```python
from build123d import *

# Parameters (mm, degrees)
PAD001_DEPTH         = 8
SKETCH004_R          = 1.6
POCKET001_DEPTH      = 5.301
POCKET001_DEPTH_BACK = 3.3011
SKETCH_W             = 17.3
SKETCH_H             = 12
SKETCH_R             = 1.5
SKETCH_R_2           = 1.6
PAD_DEPTH            = 5
SKETCH001_W          = 14
SKETCH001_H          = 12
SKETCH001_R          = 2.5
SKETCH001_R_2        = 1
POCKET_DEPTH         = 3.001
FILLET_R             = 3


with BuildPart() as clipbody:
    # Sketch003 → Pad001 (new body)
    with BuildSketch(Plane.XZ):
        with BuildLine():
            Line((0, -5.3), (-12, -5.3))
            Line((-12, -2.8), (-12, -5.3))
            Line((-1.746425, -2.8), (-12, -2.8))
            ThreePointArc((-1.746425, -2.8), (3.3, 0), (-1.746425, 2.8))
            Line((-1.746425, 2.8), (-12, 2.8))
            Line((-12, 2.8), (-12, 3.3001))
            Line((5.3, 3.3001), (-12, 3.3001))
            Line((5.3, 0), (5.3, 3.3001))
            ThreePointArc((0, -5.3), (3.747666, -3.747666), (5.3, 0))
        make_face()
    extrude(amount=-PAD001_DEPTH)

    # Sketch004 → Pocket001 (cut, two sides)
    with BuildSketch(Plane.XY) as pocket001_sk:
        with Locations((-9.5, 4)):
            Circle(SKETCH004_R)
    extrude(amount=-POCKET001_DEPTH, mode=Mode.SUBTRACT)
    extrude(pocket001_sk.sketch, amount=POCKET001_DEPTH_BACK, mode=Mode.SUBTRACT)


with BuildPart() as part_refined:
    # Sketch → Pad (new body)
    with BuildSketch(Plane.XY):
        with Locations((8.65, 6)):
            Rectangle(SKETCH_W, SKETCH_H)
        with Locations((9, 6)):
            Circle(SKETCH_R, mode=Mode.SUBTRACT)
        with Locations((2.5, 4)):
            Circle(SKETCH_R_2, mode=Mode.SUBTRACT)
    extrude(amount=PAD_DEPTH)

    # Sketch001 (on DatumPlane) → Pocket (cut, through all)
    with BuildSketch(Plane.XY.offset(2)):
        with Locations((12, 6)):
            Rectangle(SKETCH001_W, SKETCH001_H)
        with Locations((9, 6)):
            Circle(SKETCH001_R, mode=Mode.SUBTRACT)
        with Locations((14, 9.1)):
            Circle(SKETCH001_R_2, mode=Mode.SUBTRACT)
        with Locations((14, 2.9)):
            Circle(SKETCH001_R_2, mode=Mode.SUBTRACT)
    extrude(amount=POCKET_DEPTH, mode=Mode.SUBTRACT)

    # Fillet
    fillet_edges = [part_refined.edges().sort_by_distance(p)[0] for p in [
        (17.3, 12, 1),
    ]]
    fillet(fillet_edges, radius=FILLET_R)


with BuildPart() as part_refined_1:
    # Body placement: moved
    add(part_refined.part.moved(Location((-12, 0, 3.3))))

    # Fusion: union ClipBody
    add(clipbody.part)


solid = part_refined_1.part
```
Part model, mm, in its own coordinate system. A direction names the side the tool comes from. Coordinates: 2 decimals unless noted, no trailing zeros. Order: outer loops, then holes, each group sorted by start corner. A loop starts at its lowest first (then second) coordinate and runs counter-clockwise, first axis right, second up. Notation, with made-up numbers: (39, 83.25) - (96, 83.25) arc R29 ccw to (96, 115.25) - close; hole circle Ø7 at (46, 4.25). An arc over 180 degrees is marked (long way). Return JSON: item names as keys, results as strings. Group by question number.
Item 1: Cut at B-B (z = 5.75). List the corners of the cut face in (x, y), plus the area to 3 significant figures.
Item 2: Cut at A-A (x = -3). List the corners of the cut face in (y, z).
Item 3: Cut at C-C (x = -9.5). List the corners of the cut face in (y, z).
Item 4: Pin check, flat tips, straight feed: pin 1 (1.5 mm diameter, centred on x = -4.5, z = 6.5, fed in from +Y); pin 2 (0.9 mm diameter, centred on y = 7.5, z = 7, fed in from +X); pin 3 (1.5 mm diameter, centred on x = -3.5, y = 5.5, fed in from +Z); pin 4 (2.5 mm diameter, centred on x = -9.5, y = 4, fed in from +Z). Stop position of each tip, or through.
Item 5: Drill centre lines: probe 1 along Y at (x, z) = (-3, 6.65); probe 2 along Y at (x, z) = (-9.5, -4.15); probe 3 along Z at (x, y) = (0, 6). Where is each one in solid material? Low to high. Write a range as from..to.
Item 6: Which spindle directions (+Z, -Z, +X, -X, +Y, -Y) get a long thin tool onto all of the face, cutting with end or side? Do faces 4 (the face through (-3.33, 8.48, 6.78)), 5 (the face through (-7, 4, -2.8)), 6 (the face through (-7, 6, 7)). Say none if no direction does.
Item 7: Cut at D-D (y = 6.5). List the corners of the cut face in (x, z), plus the area to 3 significant figures.
Item 8: Pull direction X, two halves, no side cores. Call faces 1 (the face through (-3, 10, 3.3)), 2 (the face through (-3, 6, 3.3)), 3 (the face through (-12, 6, 6)): pulls with the +X half, pulls with the -X half, needs draft (parallel to the pull), parting line crosses it, or undercut.
Check values:
{
 "1": {"outline": "(-12, 0) - (-7, 0) - (-7, 12) - (-12, 12) - close; circle Ø5 at (-3, 6); circle Ø2 at (2, 2.9); circle Ø2 at (2, 9.1); hole circle Ø3.2 at (-9.5, 4); hole circle Ø3 at (-3, 6)", "area": "70.8 mm2"},
 "2": {"outline": "(0, -5.3) - (8, -5.3) - (8, -2.8) - (0, -2.8) - close; (0, 2.8) - (8, 2.8) - (8, 3.3) - (12, 3.3) - (12, 5.3) - (8.5, 5.3) - (8.5, 8.3) - (7.5, 8.3) - (7.5, 3.3) - (4.5, 3.3) - (4.5, 8.3) - (3.5, 8.3) - (3.5, 5.3) - (0, 5.3) - close"},
 "3": {"outline": "(0, -5.3) - (2.4, -5.3) - (2.4, -2.8) - (0, -2.8) - close; (0, 2.8) - (2.4, 2.8) - (2.4, 8.3) - (0, 8.3) - close; (5.6, -5.3) - (8, -5.3) - (8, -2.8) - (5.6, -2.8) - close; (5.6, 2.8) - (8, 2.8) - (8, 3.3) - (12, 3.3) - (12, 8.3) - (5.6, 8.3) - close"},
 "4": {"pin 1": "stops at y = 8.38", "pin 2": "stops at x = -0.73", "pin 3": "stops at z = 3.3", "pin 4": "passes through"},
 "5": {"probe 1": "y = 3.5..4.5, 7.5..8.5", "probe 2": "y = 0..2.4, 5.6..8", "probe 3": "z = -5.3..-3.3, 3.3..5.3"},
 "6": {"face 4": "+Z", "face 5": "-X, +Y, -Y", "face 6": "+Z, +Y, -Y"},
 "7": {"outline": "(-12, -5.3) - (0, -5.3) arc R5.3 ccw to (5.3, 0) - (5.3, 5.3) - (-0.55, 5.3) - (-0.55, 8.3) - (-1.59, 8.3) - (-1.59, 3.3) - (-4.41, 3.3) - (-4.41, 8.3) - (-5.45, 8.3) - (-5.45, 5.3) - (-7, 5.3) - (-7, 8.3) - (-12, 8.3) - (-12, 2.8) - (-1.75, 2.8) arc R3.3 cw (long way) to (-1.75, -2.8) - (-12, -2.8) - close", "area": "107 mm2"},
 "8": {"face 1": "needs draft", "face 2": "undercut", "face 3": "pulls with the -X half"}
}
